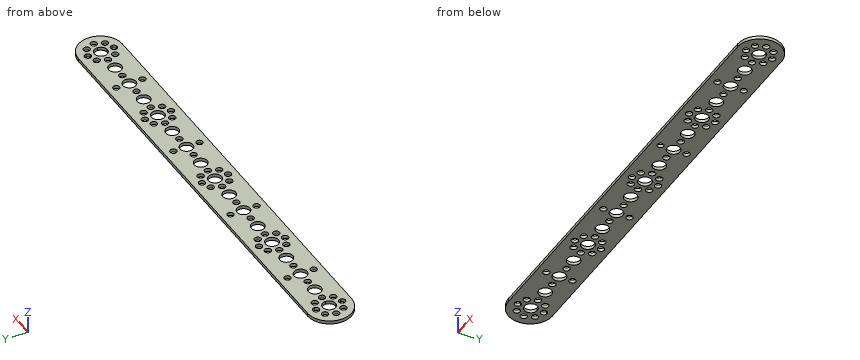
```python
from build123d import *

# Parameters (mm, degrees)
F0_R     = 2
F0_R_2   = 4
F1_DEPTH = 2


with BuildPart() as f1:
    # F0 (on Top) → F1 (new body)
    with BuildSketch(Plane.XY):
        with BuildLine():
            Line((128.5, 9.936492), (128.5, 13.5))
            Line((128.5, 13.5), (-128.5, 13.5))
            Line((-128.5, 13.5), (-128.5, 9.936492))
            ThreePointArc((-128.5, 9.936492), (-126.775255, 9.581139), (-126, 8))
            ThreePointArc((-126, 8), (-126.775255, 6.418861), (-128.5, 6.063508))
            Line((-128.5, 6.063508), (-128.5, 3.968627))
            ThreePointArc((-128.5, 3.968627), (-125.354249, 3), (-124, 0))
            ThreePointArc((-124, 0), (-125.354249, -3), (-128.5, -3.968627))
            Line((-128.5, -3.968627), (-128.5, -6.063508))
            ThreePointArc((-128.5, -6.063508), (-126.775255, -6.418861), (-126, -8))
            ThreePointArc((-126, -8), (-126.775255, -9.581139), (-128.5, -9.936492))
            Line((-128.5, -9.936492), (-128.5, -13.5))
            Line((-128.5, -13.5), (128.5, -13.5))
            Line((128.5, -13.5), (128.5, -9.936492))
            ThreePointArc((128.5, -9.936492), (126, -8), (128.5, -6.063508))
            Line((128.5, -6.063508), (128.5, -3.968627))
            ThreePointArc((128.5, -3.968627), (124, 0), (128.5, 3.968627))
            Line((128.5, 3.968627), (128.5, 6.063508))
            ThreePointArc((128.5, 6.063508), (126, 8), (128.5, 9.936492))
        make_face()
        with Locations((-96, -8)):
            Circle(F0_R, mode=Mode.SUBTRACT)
        with Locations((-64, -8)):
            Circle(F0_R, mode=Mode.SUBTRACT)
        with Locations((-32, -8)):
            Circle(F0_R, mode=Mode.SUBTRACT)
        with Locations((-122.343146, -5.656854)):
            Circle(F0_R, mode=Mode.SUBTRACT)
        with Locations((-69.656854, -5.656854)):
            Circle(F0_R, mode=Mode.SUBTRACT)
        with Locations((-58.343146, -5.656854)):
            Circle(F0_R, mode=Mode.SUBTRACT)
        with Locations((-5.656854, -5.656854)):
            Circle(F0_R, mode=Mode.SUBTRACT)
        with Locations((0, -8)):
            Circle(F0_R, mode=Mode.SUBTRACT)
        with Locations((32, -8)):
            Circle(F0_R, mode=Mode.SUBTRACT)
        with Locations((64, -8)):
            Circle(F0_R, mode=Mode.SUBTRACT)
        with Locations((96, -8)):
            Circle(F0_R, mode=Mode.SUBTRACT)
        with Locations((5.656854, -5.656854)):
            Circle(F0_R, mode=Mode.SUBTRACT)
        with Locations((58.343146, -5.656854)):
            Circle(F0_R, mode=Mode.SUBTRACT)
        with Locations((69.656854, -5.656854)):
            Circle(F0_R, mode=Mode.SUBTRACT)
        with Locations((122.343146, -5.656854)):
            Circle(F0_R, mode=Mode.SUBTRACT)
        with Locations((-120, 0)):
            Circle(F0_R, mode=Mode.SUBTRACT)
        with Locations((-112, 0)):
            Circle(F0_R_2, mode=Mode.SUBTRACT)
        with Locations((-104, 0)):
            Circle(F0_R, mode=Mode.SUBTRACT)
        with Locations((-96, 0)):
            Circle(F0_R_2, mode=Mode.SUBTRACT)
        with Locations((-88, 0)):
            Circle(F0_R, mode=Mode.SUBTRACT)
        with Locations((-80, 0)):
            Circle(F0_R_2, mode=Mode.SUBTRACT)
        with Locations((-72, 0)):
            Circle(F0_R, mode=Mode.SUBTRACT)
        with Locations((-122.343146, 5.656854)):
            Circle(F0_R, mode=Mode.SUBTRACT)
        with Locations((-64, 0)):
            Circle(F0_R_2, mode=Mode.SUBTRACT)
        with Locations((-56, 0)):
            Circle(F0_R, mode=Mode.SUBTRACT)
        with Locations((-48, 0)):
            Circle(F0_R_2, mode=Mode.SUBTRACT)
        with Locations((-40, 0)):
            Circle(F0_R, mode=Mode.SUBTRACT)
        with Locations((-32, 0)):
            Circle(F0_R_2, mode=Mode.SUBTRACT)
        with Locations((-24, 0)):
            Circle(F0_R, mode=Mode.SUBTRACT)
        with Locations((-16, 0)):
            Circle(F0_R_2, mode=Mode.SUBTRACT)
        with Locations((-8, 0)):
            Circle(F0_R, mode=Mode.SUBTRACT)
        with Locations((-69.656854, 5.656854)):
            Circle(F0_R, mode=Mode.SUBTRACT)
        with Locations((-58.343146, 5.656854)):
            Circle(F0_R, mode=Mode.SUBTRACT)
        with Locations((-5.656854, 5.656854)):
            Circle(F0_R, mode=Mode.SUBTRACT)
        with Locations((-96, 8)):
            Circle(F0_R, mode=Mode.SUBTRACT)
        with Locations((-64, 8)):
            Circle(F0_R, mode=Mode.SUBTRACT)
        with Locations((-32, 8)):
            Circle(F0_R, mode=Mode.SUBTRACT)
        Circle(F0_R_2, mode=Mode.SUBTRACT)
        with Locations((8, 0)):
            Circle(F0_R, mode=Mode.SUBTRACT)
        with Locations((16, 0)):
            Circle(F0_R_2, mode=Mode.SUBTRACT)
        with Locations((24, 0)):
            Circle(F0_R, mode=Mode.SUBTRACT)
        with Locations((32, 0)):
            Circle(F0_R_2, mode=Mode.SUBTRACT)
        with Locations((40, 0)):
            Circle(F0_R, mode=Mode.SUBTRACT)
        with Locations((48, 0)):
            Circle(F0_R_2, mode=Mode.SUBTRACT)
        with Locations((56, 0)):
            Circle(F0_R, mode=Mode.SUBTRACT)
        with Locations((64, 0)):
            Circle(F0_R_2, mode=Mode.SUBTRACT)
        with Locations((5.656854, 5.656854)):
            Circle(F0_R, mode=Mode.SUBTRACT)
        with Locations((58.343146, 5.656854)):
            Circle(F0_R, mode=Mode.SUBTRACT)
        with Locations((69.656854, 5.656854)):
            Circle(F0_R, mode=Mode.SUBTRACT)
        with Locations((72, 0)):
            Circle(F0_R, mode=Mode.SUBTRACT)
        with Locations((80, 0)):
            Circle(F0_R_2, mode=Mode.SUBTRACT)
        with Locations((88, 0)):
            Circle(F0_R, mode=Mode.SUBTRACT)
        with Locations((96, 0)):
            Circle(F0_R_2, mode=Mode.SUBTRACT)
        with Locations((104, 0)):
            Circle(F0_R, mode=Mode.SUBTRACT)
        with Locations((112, 0)):
            Circle(F0_R_2, mode=Mode.SUBTRACT)
        with Locations((120, 0)):
            Circle(F0_R, mode=Mode.SUBTRACT)
        with Locations((122.343146, 5.656854)):
            Circle(F0_R, mode=Mode.SUBTRACT)
        with Locations((0, 8)):
            Circle(F0_R, mode=Mode.SUBTRACT)
        with Locations((32, 8)):
            Circle(F0_R, mode=Mode.SUBTRACT)
        with Locations((64, 8)):
            Circle(F0_R, mode=Mode.SUBTRACT)
        with Locations((96, 8)):
            Circle(F0_R, mode=Mode.SUBTRACT)
        with BuildLine():
            Line((-128.5, 9.936492), (-128.5, 13.5))
            ThreePointArc((-128.5, 13.5), (-142, 0), (-128.5, -13.5))
            Line((-128.5, -13.5), (-128.5, -9.936492))
            ThreePointArc((-128.5, -9.936492), (-130, -8), (-128.5, -6.063508))
            Line((-128.5, -6.063508), (-128.5, -3.968627))
            ThreePointArc((-128.5, -3.968627), (-132, 0), (-128.5, 3.968627))
            Line((-128.5, 3.968627), (-128.5, 6.063508))
            ThreePointArc((-128.5, 6.063508), (-130, 8), (-128.5, 9.936492))
        make_face()
        with Locations((-133.656854, -5.656854)):
            Circle(F0_R, mode=Mode.SUBTRACT)
        with Locations((-136, 0)):
            Circle(F0_R, mode=Mode.SUBTRACT)
        with Locations((-133.656854, 5.656854)):
            Circle(F0_R, mode=Mode.SUBTRACT)
        with BuildLine():
            ThreePointArc((128.5, -13.5), (142, 0), (128.5, 13.5))
            Line((128.5, 13.5), (128.5, 9.936492))
            ThreePointArc((128.5, 9.936492), (129.581139, 9.224745), (130, 8))
            ThreePointArc((130, 8), (129.581139, 6.775255), (128.5, 6.063508))
            Line((128.5, 6.063508), (128.5, 3.968627))
            ThreePointArc((128.5, 3.968627), (131, 2.645751), (132, 0))
            ThreePointArc((132, 0), (131, -2.645751), (128.5, -3.968627))
            Line((128.5, -3.968627), (128.5, -6.063508))
            ThreePointArc((128.5, -6.063508), (129.581139, -6.775255), (130, -8))
            ThreePointArc((130, -8), (129.581139, -9.224745), (128.5, -9.936492))
            Line((128.5, -9.936492), (128.5, -13.5))
        make_face()
        with Locations((133.656854, -5.656854)):
            Circle(F0_R, mode=Mode.SUBTRACT)
        with Locations((136, 0)):
            Circle(F0_R, mode=Mode.SUBTRACT)
        with Locations((133.656854, 5.656854)):
            Circle(F0_R, mode=Mode.SUBTRACT)
    extrude(amount=F1_DEPTH)


solid = f1.part
```
Verification items for the finished model (mm, model axes). Coordinates: 2 decimals unless noted, no trailing zeros. Loops run counter-clockwise (first coordinate to the right, second up) from the corner with the lowest first, then second, coordinate; pieces in that order, holes last. Notation, with made-up numbers: (29.25, 53.5) -> (71.25, 53.5) arc R32 cw to (71.25, 88.5) -> close; hole circle Ø9 at (60, 87.25). An arc over 180 degrees is marked (long way). Answer in a Markdown table with one row per item.
1) Section check B-B (z = 1.5). Give the number of separate pieces and of enclosed holes in the cut face, and give its area (3 significant figures).
The answers:
| item | result |
|---|---|
| separate pieces | 1 |
| enclosed holes | 73 |
| area | 5,950 mm2 |
2) Scan lines: line 1 along Y through (x, z) = (40, 0.8); line 2 along Y through (x, z) = (40.5, 1.2); line 3 along Y through (x, z) = (4.5, 1.75). Record each from-to range of solid material in increasing order. Write a range as from..to.
The answers:
| item | result |
|---|---|
| line 1 | y = -13.5..-2, 2..13.5 |
| line 2 | y = -13.5..-1.94, 1.94..13.5 |
| line 3 | y = -13.5..-7.29, -4.03..4.03, 7.29..13.5 |
3) Depth check by flat-ended pin: P1, Ø5, axis at x = -96, y = 8, coming from the -Z side; P2, Ø3, axis at x = -32, y = -8, coming from the +Z side. Enter the tip coordinate at first touch or a pass-through.
The answers:
| item | result |
|---|---|
| P1 | stops at z = 0 |
| P2 | passes through |
4) Section check A-A (x = -16). Record the cut outline in (y, z), and give its area (3 significant figures).
The answers:
| item | result |
|---|---|
| outline | (-13.5, 0) -> (-4, 0) -> (-4, 2) -> (-13.5, 2) -> close; (4, 0) -> (13.5, 0) -> (13.5, 2) -> (4, 2) -> close |
| area | 38.0 mm2 |
